from build123d import *

# Parameters (mm, degrees)
SKETCH1_R               = 2.5
BOSS_EXTRUDE1_DEPTH     = 150
SKETCH2_R               = 3.75
BOSS_EXTRUDE2_DEPTH     = 3
FILLET1_R               = 1
CUT_EXTRUDE1_DEPTH      = 10
CUT_EXTRUDE1_DEPTH_BACK = 10
FILLET2_R               = 0.5


with BuildPart() as part:
    # Sketch1 → Boss-Extrude1 (new body)
    with BuildSketch(Plane(origin=(0, 0, 0), x_dir=(1, 0, 0), z_dir=(0, 1, 0))):
        Circle(SKETCH1_R)
    extrude(amount=BOSS_EXTRUDE1_DEPTH)

    # Sketch2 → Boss-Extrude2 (add)
    with BuildSketch(Plane(origin=(0, 150, 0), x_dir=(1, 0, 0), z_dir=(0, 1, 0))):
        Circle(SKETCH2_R)
    extrude(amount=BOSS_EXTRUDE2_DEPTH)

    # Fillet1
    fillet1_edges = [part.edges().sort_by_distance(p)[0] for p in [
        (-3.75, 153, 0),
    ]]
    fillet(fillet1_edges, radius=FILLET1_R)

    # Sketch4 → Cut-Extrude1 (cut, two sides)
    with BuildSketch(Plane.XY) as cut_extrude1_sk:
        Polygon((0, 152), (-0.577350269, 153), (0.577350269, 153), align=None)
    extrude(amount=CUT_EXTRUDE1_DEPTH, mode=Mode.SUBTRACT)
    extrude(cut_extrude1_sk.sketch, amount=-CUT_EXTRUDE1_DEPTH_BACK, mode=Mode.SUBTRACT)

    # Fillet2
    fillet2_edges = [part.edges().sort_by_distance(p)[0] for p in [
        (-3.75, 150, 0),
    ]]
    fillet(fillet2_edges, radius=FILLET2_R)


solid = part.part
Could you check a few things on this model? Use its own coordinates, in mm. A direction names the side the tool comes from. Coordinates: 2 decimals unless noted, no trailing zeros. Write each loop counter-clockwise with the first axis right and the second up, starting at its lowest first coordinate (ties: lowest second). Pieces come first, ordered by that corner, then holes. Notation, with made-up numbers: M 20.5,72 L 52.5,72 A18 cw 52.5,76 Z; hole C 35.25,-8.5 d7. An arc over 180 degrees is marked long. One line per question, with ' | ' between items.
1) For faces 1 (the face through (-0.54, 73.95, 2.44)), 2 (the face through (0, 0, 0)), which set-ups out of +Z, -Z, +X, -X, +Y, -Y let a thin tool reach every point of the face, with its end or its side?
Checks:
face 1: -Y | face 2: +Z, -Z, +X, -X, -Y
2) Imagine slicing it at B-B, the plane y = 50.5. Write out the boundary of the cut face in (x, z).
Checks:
outline: C 0,0 d5
3) For pin 1 Ø4 at (y, z) = (47.5, 2.5) entering from -X; pin 2 Ø1 at (y, z) = (85.5, -0.5) entering from -X; pin 3 Ø1.5 at (y, z) = (105, -1.5) entering from +X, each with a flat end and sliding along its axis, tell me the tip position at first contact or that it passes through.
Checks:
pin 1: x = -2.45 | pin 2: x = -2.5 | pin 3: x = 2.38
4) I need wall thicknesses on probe 1 along Y at (x, z) = (-2, 1.75); probe 2 along Z at (x, y) = (0.25, 57.5). Which ranges of each line are inside material? Lowest first, please. Write a range as [from, to].
Checks:
probe 1: [150, 153] | probe 2: [-2.49, 2.49]
5) Imagine slicing it at A-A, the plane z = 0. Write out the boundary of the cut face in (x, y), and give its area (3 significant figures).
Checks:
outline: M -3.75,150.5 A0.5 ccw -3.25,150 L -2.5,150 L -2.5,0 L 2.5,0 L 2.5,150 L 3.25,150 A0.5 ccw 3.75,150.5 L 3.75,152 A1 ccw 2.75,153 L 0.58,153 L 0,152 L -0.58,153 L -2.75,153 A1 ccw -3.75,152 Z | area: 771 mm²
